Check sheet for the modelled part. Datum: model origin and axes. Units: mm. A direction names the side the tool comes from. Coordinates: 2 decimals unless noted, no trailing zeros. Loops run counter-clockwise (first coordinate to the right, second up) from the corner with the lowest first, then second, coordinate; pieces in that order, holes last.
```python
from build123d import *

# Parameters (mm, degrees)
SKETCH2_W           = 54
SKETCH2_H           = 123
SKETCH2_W_2         = 32
SKETCH2_H_2         = 100
SKETCH12_W          = 54
SKETCH12_H          = 123
SKETCH12_W_2        = 32
SKETCH12_H_2        = 100
BOSS_EXTRUDE1_DEPTH = 1
SKETCH3_W           = 54
SKETCH3_H           = 127
SKETCH3_W_2         = 32
SKETCH3_H_2         = 100
EXTRUDE1_DEPTH      = 73
EXTRUDE2_START      = -54
SKETCH4_R           = 2.75
SKETCH4_W           = 100
SKETCH4_H           = 50
EXTRUDE2_DEPTH      = 54
SKETCH7_W           = 54
SKETCH7_H           = 127
SKETCH7_W_2         = 32
SKETCH7_H_2         = 100
EXTRUDE5_DEPTH      = 73
EXTRUDE6_REACH      = 1082.845
SKETCH8_R           = 2.75
SKETCH8_W           = 100
SKETCH8_H           = 50
SKETCH5_W           = 42
SKETCH5_H           = 36.5
EXTRUDE3_DEPTH      = 11.5
SKETCH6_W           = 42
SKETCH6_H           = 36.5
EXTRUDE4_DEPTH      = 11.5
SKETCH9_R           = 2.75
EXTRUDE7_DEPTH      = 7
SKETCH10_R          = 2.75
EXTRUDE8_DEPTH      = 7


with BuildPart() as part:
    # Sweep1: sweep along a path in Sketch1
    with BuildLine(Plane.XY) as sweep1_path:
        Line((-311.2, 954.5), (-311.2, 904.5))
        ThreePointArc((-311.2, 904.5), (-311.146227919, 900.833921861), (-310.984957937, 897.170997845))
        Line((-310.984957937, 897.170997845), (-249.784957937, -144.831619147))
        ThreePointArc((-249.784957937, -144.831619147), (-121.333921861, -262.44884491), (0, -137.502616992))
        Line((0, -137.502616992), (0, 0))
    # Sketch2 → Sweep1 (sweep)
    with BuildSketch(Plane(origin=(0, 0, 0), x_dir=(1, 0, 0), z_dir=(0, 1, 0))):
        with Locations((0, -61.5)):
            Rectangle(SKETCH2_W, SKETCH2_H)
        with Locations((0, -61.5)):
            Rectangle(SKETCH2_W_2, SKETCH2_H_2, mode=Mode.SUBTRACT)
    sweep(path=sweep1_path.line)

    # Sketch12 → Boss-Extrude1 (add)
    with BuildSketch(Plane(origin=(0, 0, 0), x_dir=(1, 0, 0), z_dir=(0, 1, 0))):
        with Locations((0, -61.5)):
            Rectangle(SKETCH12_W, SKETCH12_H)
        with Locations((0, -61.5)):
            Rectangle(SKETCH12_W_2, SKETCH12_H_2, mode=Mode.SUBTRACT)
    extrude(amount=BOSS_EXTRUDE1_DEPTH)

    # Sketch3 → Extrude1 (add)
    with BuildSketch(Plane(origin=(0, 1, 0), x_dir=(1, 0, 0), z_dir=(0, 1, 0))):
        with Locations((0, -61.5)):
            Rectangle(SKETCH3_W, SKETCH3_H)
        with Locations((0, -61.5)):
            Rectangle(SKETCH3_W_2, SKETCH3_H_2, mode=Mode.SUBTRACT)
    extrude(amount=EXTRUDE1_DEPTH)

    # Sketch4 → Extrude2 (cut)
    with BuildSketch(Plane(origin=(27, 0, 0), x_dir=(0, 0, -1), z_dir=(1, 0, 0)).offset(EXTRUDE2_START)):
        with Locations((-118.5, 61.5)):
            Circle(SKETCH4_R)
        with Locations((-118.5, 39)):
            Circle(SKETCH4_R)
        with Locations((-4.5, 39)):
            Circle(SKETCH4_R)
        with Locations((-4.5, 61.5)):
            Circle(SKETCH4_R)
        with Locations((-61.5, 49)):
            Rectangle(SKETCH4_W, SKETCH4_H)
    extrude(amount=EXTRUDE2_DEPTH, mode=Mode.SUBTRACT)

    # Sketch7 → Extrude5 (add)
    with BuildSketch(Plane(origin=(0, 954.5, 0), x_dir=(1, 0, 0), z_dir=(0, 1, 0))):
        with Locations((-311.2, -61.5)):
            Rectangle(SKETCH7_W, SKETCH7_H)
        with Locations((-311.2, -61.5)):
            Rectangle(SKETCH7_W_2, SKETCH7_H_2, mode=Mode.SUBTRACT)
    extrude(amount=EXTRUDE5_DEPTH)

    # Extrude6: up to this face of the body (flat: up to its plane)
    extrude6_end = Plane(part.part.faces().sort_by_distance((-338.2, 966.473380455, 61.5))[0])
    # Sketch8 → Extrude6 (cut, up to the picked face)
    with BuildSketch(Plane(origin=(-284.2, 0, 0), x_dir=(0, 0, -1), z_dir=(1, 0, 0)), mode=Mode.PRIVATE) as extrude6_sk1:
        with Locations((-4.5, 992.5)):
            Circle(SKETCH8_R)
    extrude6_tool1 = split(extrude(extrude6_sk1.sketch, amount=-EXTRUDE6_REACH, mode=Mode.PRIVATE), bisect_by=extrude6_end, keep=Keep.BOTH, mode=Mode.PRIVATE)
    # Sketch8 → Extrude6 (cut, up to the picked face)
    with BuildSketch(Plane(origin=(-284.2, 0, 0), x_dir=(0, 0, -1), z_dir=(1, 0, 0)), mode=Mode.PRIVATE) as extrude6_sk2:
        with Locations((-4.5, 1015)):
            Circle(SKETCH8_R)
    extrude6_tool2 = split(extrude(extrude6_sk2.sketch, amount=-EXTRUDE6_REACH, mode=Mode.PRIVATE), bisect_by=extrude6_end, keep=Keep.BOTH, mode=Mode.PRIVATE)
    # Sketch8 → Extrude6 (cut, up to the picked face)
    with BuildSketch(Plane(origin=(-284.2, 0, 0), x_dir=(0, 0, -1), z_dir=(1, 0, 0)), mode=Mode.PRIVATE) as extrude6_sk3:
        with Locations((-118.5, 992.5)):
            Circle(SKETCH8_R)
    extrude6_tool3 = split(extrude(extrude6_sk3.sketch, amount=-EXTRUDE6_REACH, mode=Mode.PRIVATE), bisect_by=extrude6_end, keep=Keep.BOTH, mode=Mode.PRIVATE)
    # Sketch8 → Extrude6 (cut, up to the picked face)
    with BuildSketch(Plane(origin=(-284.2, 0, 0), x_dir=(0, 0, -1), z_dir=(1, 0, 0)), mode=Mode.PRIVATE) as extrude6_sk4:
        with Locations((-118.5, 1015)):
            Circle(SKETCH8_R)
    extrude6_tool4 = split(extrude(extrude6_sk4.sketch, amount=-EXTRUDE6_REACH, mode=Mode.PRIVATE), bisect_by=extrude6_end, keep=Keep.BOTH, mode=Mode.PRIVATE)
    # Sketch8 → Extrude6 (cut, up to the picked face)
    with BuildSketch(Plane(origin=(-284.2, 0, 0), x_dir=(0, 0, -1), z_dir=(1, 0, 0)), mode=Mode.PRIVATE) as extrude6_sk5:
        with Locations((-61.5, 1002.5)):
            Rectangle(SKETCH8_W, SKETCH8_H)
    extrude6_tool5 = split(extrude(extrude6_sk5.sketch, amount=-EXTRUDE6_REACH, mode=Mode.PRIVATE), bisect_by=extrude6_end, keep=Keep.BOTH, mode=Mode.PRIVATE)
    add(extrude6_tool1.solids().sort_by(Axis((-284.2, 992.5, 4.5), (-1, 0, 0)))[0], mode=Mode.SUBTRACT)
    add(extrude6_tool2.solids().sort_by(Axis((-284.2, 1015, 4.5), (-1, 0, 0)))[0], mode=Mode.SUBTRACT)
    add(extrude6_tool3.solids().sort_by(Axis((-284.2, 992.5, 118.5), (-1, 0, 0)))[0], mode=Mode.SUBTRACT)
    add(extrude6_tool4.solids().sort_by(Axis((-284.2, 1015, 118.5), (-1, 0, 0)))[0], mode=Mode.SUBTRACT)
    add(extrude6_tool5.solids().sort_by(Axis((-284.2, 1002.5, 61.5), (-1, 0, 0)))[0], mode=Mode.SUBTRACT)

    # Sketch5 → Extrude3 (cut)
    with BuildSketch(Plane.XY.offset(125)):
        with Locations((0, 49.75)):
            Rectangle(SKETCH5_W, SKETCH5_H)
        with Locations((-311.2, 1003.25)):
            Rectangle(SKETCH5_W, SKETCH5_H)
    extrude(amount=-EXTRUDE3_DEPTH, mode=Mode.SUBTRACT)

    # Sketch6 → Extrude4 (cut)
    with BuildSketch(Plane(origin=(0, 0, -2), x_dir=(-1, 0, 0), z_dir=(0, 0, -1))):
        with Locations((0, 49.75)):
            Rectangle(SKETCH6_W, SKETCH6_H)
        with Locations((311.2, 1003.25)):
            Rectangle(SKETCH6_W, SKETCH6_H)
    extrude(amount=-EXTRUDE4_DEPTH, mode=Mode.SUBTRACT)

    # Sketch9 → Extrude7 (cut)
    with BuildSketch(Plane(origin=(0, 74, 0), x_dir=(1, 0, 0), z_dir=(0, 1, 0))):
        with Locations(Location((-11, -118.5, 0), (0, 0, 180))):
            Circle(SKETCH9_R)
        with Locations(Location((11, -118.5, 0), (0, 0, 180))):
            Circle(SKETCH9_R)
        with Locations(Location((11, -4.5, 0), (0, 0, 180))):
            Circle(SKETCH9_R)
        with Locations(Location((-11, -4.5, 0), (0, 0, 180))):
            Circle(SKETCH9_R)
    extrude(amount=-EXTRUDE7_DEPTH, mode=Mode.SUBTRACT)

    # Sketch10 → Extrude8 (cut)
    with BuildSketch(Plane(origin=(0, 1027.5, 0), x_dir=(1, 0, 0), z_dir=(0, 1, 0))):
        with Locations(Location((-322.2, -118.5, 0), (0, 0, 270))):
            Circle(SKETCH10_R)
        with Locations(Location((-300.2, -118.5, 0), (0, 0, 270))):
            Circle(SKETCH10_R)
        with Locations(Location((-322.2, -4.5, 0), (0, 0, 270))):
            Circle(SKETCH10_R)
        with Locations(Location((-300.2, -4.5, 0), (0, 0, 270))):
            Circle(SKETCH10_R)
    extrude(amount=-EXTRUDE8_DEPTH, mode=Mode.SUBTRACT)


solid = part.part
```
1) Section check A-A on z = 65. Enter the section's corners in (x, y).
Answer sheet:
outline: (-338.2, 904.5) arc R152 ccw to (-337.94, 895.59) - (-276.74, -146.41) arc R152 ccw to (27, -137.5) - (27, 24) - (16, 24) - (16, -137.5) arc R141 cw to (-265.76, -145.77) - (-326.96, 896.23) arc R141 cw to (-327.2, 904.5) - (-327.2, 977.5) - (-338.2, 977.5) - close; (-295.2, 904.5) arc R109 ccw to (-295.01, 898.11) - (-233.81, -143.89) arc R109 ccw to (-16, -137.5) - (-16, 24) - (-27, 24) - (-27, -137.5) arc R98 cw to (-222.83, -143.25) - (-284.03, 898.75) arc R98 cw to (-284.2, 904.5) - (-284.2, 977.5) - (-295.2, 977.5) - close
2) Depth check by flat-ended pin: pin 1 (1.5 mm diameter, centred on x = -261, y = 388, fed in from -Z); pin 2 (3.5 mm diameter, centred on y = 54, z = 4.5, fed in from -X); pin 3 (11 mm diameter, centred on x = 3.5, y = 54, fed in from -Z). Enter the tip coordinate at first touch or a pass-through.
Answer sheet:
pin 1: stops at z = 0
pin 2: stops at x = -288.61
pin 3: stops at z = 9.5
3) Scan lines: line 1 (Z direction, x = -22.4, y = 39); line 2 (X direction, y = 1023, z = 4); line 3 (X direction, y = 528, z = 32). Record each from-to range of solid material in increasing order.
Answer sheet:
line 1: z = -2 to 1.75, 7.25 to 11.5, 111.5 to 115.75, 121.25 to 125
line 2: x = -338.2 to -324.9, -319.5 to -302.9, -297.5 to -284.2
line 3: x = -316.35 to -305.33, -273.27 to -262.26
4) Set-up check for faces 4 (the flat face through (0, 50, 113.5)), 5 (the flat face through (0, 50, 9.5)), 6 (the flat face through (-263, 226, 11.5)): record each of +Z, -Z, +X, -X, +Y, -Y from which the full face is reachable in a straight line by a thin tool's end or side.
Answer sheet:
face 4: +Z
face 5: -Z
face 6: none
5) Section check D-D on y = 129. Enter the section's corners in (x, z), plus the area to 3 significant figures.
Answer sheet:
outline: (-292.91, 0) - (-238.82, 0) - (-238.82, 123) - (-292.91, 123) - close; hole (-281.9, 11.5) - (-249.84, 11.5) - (-249.84, 111.5) - (-281.9, 111.5) - close
area: 3,450 mm2
6) Section check C-C on y = -57.5. Enter the section's corners in (x, z), plus the area to 3 significant figures.
Answer sheet:
outline: (-281.96, 0) - (-227.87, 0) - (-227.87, 123) - (-281.96, 123) - close; (-27, 0) - (27, 0) - (27, 123) - (-27, 123) - close; hole (-270.94, 11.5) - (-238.89, 11.5) - (-238.89, 111.5) - (-270.94, 111.5) - close; hole (-16, 11.5) - (16, 11.5) - (16, 111.5) - (-16, 111.5) - close
area: 6,890 mm2
7) Mould release check, pull along X, two halves, no side actions. Record for faces 1 (the flat face through (-311, 1004, 113.5)), 2 (the flat face through (-284.2, 951, 62)), 3 (the flat face through (-312, 982, 125)): +X half, -X half, draft (parallel to the pull), parting line (faces both ways), or undercut.
Answer sheet:
face 1: undercut
face 2: +X half
face 3: draft
8) Section check B-B on x = -125. Enter the section's corners in (y, z), plus the area to 3 significant figures.
Answer sheet:
outline: (-289.5, 0) - (-235.5, 0) - (-235.5, 123) - (-289.5, 123) - close; hole (-278.5, 11.5) - (-246.5, 11.5) - (-246.5, 111.5) - (-278.5, 111.5) - close
area: 3,440 mm2
